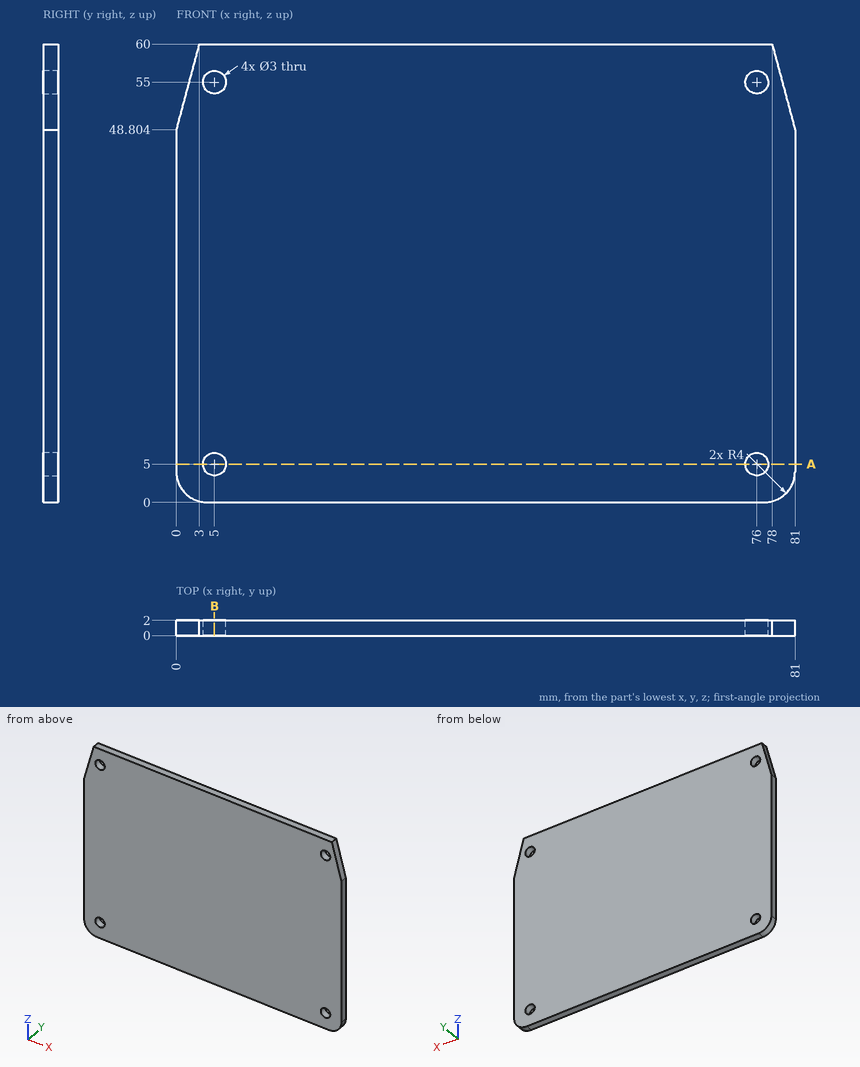
Can you work these out from the drawing? Everything is in mm from the part's minimum corner. Coordinates: 2 decimals unless noted, no trailing zeros. Write each loop counter-clockwise with the first axis right and the second up, starting at its lowest first coordinate (ties: lowest second). Pieces come first, ordered by that corner, then holes. Notation, with made-up numbers: (71, -8.5) -> (129, -8.5) arc R25 ccw to (129, 5.5) -> close; hole circle Ø9 at (-14, 71.25). An arc over 180 degrees is marked (long way). Write each question's results on one line, items separated by ' | '. Start each with the question number.
Item 1: If we section it at B-B, the plane x = 5: Write out the boundary of the cut face in (y, z), and give its area (3 significant figures).
Item 2: Please list where these lines run through material, in increasing order: probe 1 along X at (y, z) = (0.9, 5); probe 2 along Z at (x, y) = (76, 1.15); probe 3 along X at (y, z) = (0.65, 55).
Item 3: I'm going to push a flat-ended pin straight in: P1, Ø5, axis at x = 14.5, z = 16.5, coming from the -Y side. Where does the tip first touch, or does it pass through?
Item 4: If we section it at A-A, the plane z = 5: Write out the boundary of the cut face in (x, y), and give its area (3 significant figures).
Answer block:
1) outline: (0, 0) -> (2, 0) -> (2, 3.5) -> (0, 3.5) -> close; (0, 6.5) -> (2, 6.5) -> (2, 53.5) -> (0, 53.5) -> close; (0, 56.5) -> (2, 56.5) -> (2, 60) -> (0, 60) -> close | area: 108 mm²
2) probe 1: 0 to 3.5, 6.5 to 74.5, 77.5 to 81 | probe 2: 0 to 3.5, 6.5 to 53.5, 56.5 to 60 | probe 3: 1.66 to 3.5, 6.5 to 74.5, 77.5 to 79.34
3) P1: y = 0
4) outline: (0, 0) -> (3.5, 0) -> (3.5, 2) -> (0, 2) -> close; (6.5, 0) -> (74.5, 0) -> (74.5, 2) -> (6.5, 2) -> close; (77.5, 0) -> (81, 0) -> (81, 2) -> (77.5, 2) -> close | area: 150 mm²
